from build123d import *

# Parameters (mm, degrees)
BOSS_EXTRUDE1_START    = 0.03
SKETCH1_W              = 7
SKETCH1_H              = 7
BOSS_EXTRUDE1_DEPTH    = 0.73
SKETCH2_R              = 0.478943658
CUT_EXTRUDE1_DEPTH     = 0.05
BOSS_EXTRUDE2_DEPTH    = 0.03
SKETCH4_W              = 0.5
SKETCH4_H              = 0.3
BOSS_EXTRUDE3_DEPTH    = 0.03
FILLET1_R              = 0.15
LPATTERN1_COUNT        = 3
LPATTERN1_PITCH        = 1.7
FILLET1_OF_LPATTERN1_R = 0.15
CIRPATTERN1_DEPTH      = 0.03


# Read off the part's stored shape, not the designer's step: CirPattern1
with BuildPart() as part:
    # Sketch1 → Boss-Extrude1 (new body)
    with BuildSketch(Plane.XY.offset(BOSS_EXTRUDE1_START)):
        Rectangle(SKETCH1_W, SKETCH1_H)
    extrude(amount=BOSS_EXTRUDE1_DEPTH)

    # Sketch2 → Cut-Extrude1 (cut)
    with BuildSketch(Plane.XY.offset(0.76)):
        with Locations((-2.534351737, 2.640370435)):
            Circle(SKETCH2_R)
    extrude(amount=-CUT_EXTRUDE1_DEPTH, mode=Mode.SUBTRACT)

    # Sketch3 → Boss-Extrude2 (add)
    with BuildSketch(Plane(origin=(0, 0, 0.03), x_dir=(-1, 0, 0), z_dir=(0, 0, -1))):
        Polygon((1.1, 1.4), (1.4, 1.1), (1.4, -1.4), (-1.4, -1.4), (-1.4, 1.4), align=None)
    extrude(amount=BOSS_EXTRUDE2_DEPTH)

    # Sketch4 → Boss-Extrude3 (add)
    with BuildSketch(Plane(origin=(0, 0, 0.03), x_dir=(-1, 0, 0), z_dir=(0, 0, -1))):
        with Locations((-3.25, 1.7)):
            Rectangle(SKETCH4_W, SKETCH4_H)
    boss_extrude3 = extrude(amount=BOSS_EXTRUDE3_DEPTH)

    # Fillet1
    fillet1_edges = [part.edges().sort_by_distance(p)[0] for p in [
        (3, 1.85, 0.015),
        (3, 1.55, 0.015),
    ]]
    fillet(fillet1_edges, radius=FILLET1_R - 0.0001)  # a hair under: the kernel refuses the full size

    # LPattern1: Boss-Extrude3 ×3
    with Locations(*[(0, -i * LPATTERN1_PITCH, 0) for i in range(1, LPATTERN1_COUNT)]):
        add(boss_extrude3)

    # Fillet1 of LPattern1
    fillet1_of_lpattern1_edges = [part.edges().sort_by_distance(p)[0] for p in [
        (3, 0.15, 0.015),
        (3, -0.15, 0.015),
        (3, -1.55, 0.015),
        (3, -1.85, 0.015),
    ]]
    fillet(fillet1_of_lpattern1_edges, radius=FILLET1_OF_LPATTERN1_R - 0.0001)  # a hair under: the kernel refuses the full size

    # CirPattern1 outline → CirPattern1 (add)
    with BuildSketch(Plane.XY):
        with BuildLine():
            Line((-3.5, 1.85), (-3.5, 1.55))
            Line((-3.5, 1.55), (-3.15, 1.55))
            ThreePointArc((-3.15, 1.55), (-3.043933983, 1.593933983), (-3, 1.7))
            ThreePointArc((-3, 1.7), (-3.043933983, 1.806066017), (-3.15, 1.85))
            Line((-3.15, 1.85), (-3.5, 1.85))
        make_face()
        with BuildLine():
            Line((1.55, -3.15), (1.55, -3.5))
            Line((1.55, -3.5), (1.85, -3.5))
            Line((1.85, -3.5), (1.85, -3.15))
            ThreePointArc((1.85, -3.15), (1.806066017, -3.043933983), (1.7, -3))
            ThreePointArc((1.7, -3), (1.593933983, -3.043933983), (1.55, -3.15))
        make_face()
        with BuildLine():
            Line((-0.15, -3.15), (-0.15, -3.5))
            Line((-0.15, -3.5), (0.15, -3.5))
            Line((0.15, -3.5), (0.15, -3.15))
            ThreePointArc((0.15, -3.15), (0.106066017, -3.043933983), (0, -3))
            ThreePointArc((0, -3), (-0.106066017, -3.043933983), (-0.15, -3.15))
        make_face()
        with BuildLine():
            Line((-1.85, -3.15), (-1.85, -3.5))
            Line((-1.85, -3.5), (-1.55, -3.5))
            Line((-1.55, -3.5), (-1.55, -3.15))
            ThreePointArc((-1.55, -3.15), (-1.593933983, -3.043933983), (-1.7, -3))
            ThreePointArc((-1.7, -3), (-1.806066017, -3.043933983), (-1.85, -3.15))
        make_face()
        with BuildLine():
            Line((-3.15, -1.55), (-3.5, -1.55))
            Line((-3.5, -1.55), (-3.5, -1.85))
            Line((-3.5, -1.85), (-3.15, -1.85))
            ThreePointArc((-3.15, -1.85), (-3.043933983, -1.806066017), (-3, -1.7))
            ThreePointArc((-3, -1.7), (-3.043933983, -1.593933983), (-3.15, -1.55))
        make_face()
        with BuildLine():
            Line((-3.15, 0.15), (-3.5, 0.15))
            Line((-3.5, 0.15), (-3.5, -0.15))
            Line((-3.5, -0.15), (-3.15, -0.15))
            ThreePointArc((-3.15, -0.15), (-3.043933983, -0.106066017), (-3, 0))
            ThreePointArc((-3, 0), (-3.043933983, 0.106066017), (-3.15, 0.15))
        make_face()
        with BuildLine():
            Line((1.85, 3.5), (1.55, 3.5))
            Line((1.55, 3.5), (1.55, 3.15))
            ThreePointArc((1.55, 3.15), (1.593933983, 3.043933983), (1.7, 3))
            ThreePointArc((1.7, 3), (1.806066017, 3.043933983), (1.85, 3.15))
            Line((1.85, 3.15), (1.85, 3.5))
        make_face()
        with BuildLine():
            Line((0.15, 3.5), (-0.15, 3.5))
            Line((-0.15, 3.5), (-0.15, 3.15))
            ThreePointArc((-0.15, 3.15), (-0.106066017, 3.043933983), (0, 3))
            ThreePointArc((0, 3), (0.106066017, 3.043933983), (0.15, 3.15))
            Line((0.15, 3.15), (0.15, 3.5))
        make_face()
        with BuildLine():
            Line((-1.55, 3.5), (-1.85, 3.5))
            Line((-1.85, 3.5), (-1.85, 3.15))
            ThreePointArc((-1.85, 3.15), (-1.806066017, 3.043933983), (-1.7, 3))
            ThreePointArc((-1.7, 3), (-1.593933983, 3.043933983), (-1.55, 3.15))
            Line((-1.55, 3.15), (-1.55, 3.5))
        make_face()
    extrude(amount=CIRPATTERN1_DEPTH)


solid = part.part
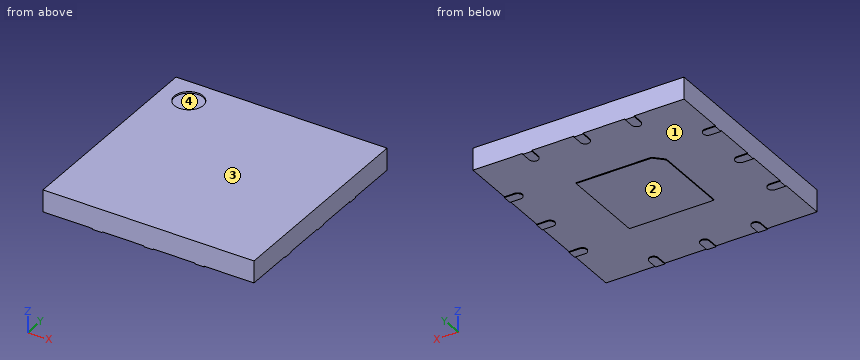
Input: part model. Units: mm. Frame: model coordinates. Face numbers are marked on the shaded views. A direction names the side the tool comes from. Coordinates: 2 decimals unless noted, no trailing zeros. Order: outer loops, then holes, each group sorted by start corner. A loop starts at its lowest first (then second) coordinate and runs counter-clockwise, first axis right, second up. Notation, with made-up numbers: M -2.5,10 L 32.5,10 A17 ccw 32.5,23 Z; hole C -28,67 d11. An arc over 180 degrees is marked long. Answer in a Markdown table with one row per item.
(1) Section query C-C, the plane x = 2. Output: boundary loops of the cut face in (y, z).
Numbers:
| item | result |
|---|---|
| outline | M -3.5,0.03 L 3.5,0.03 L 3.5,0.76 L -3.5,0.76 Z |
(2) Material intervals for line 1 (Z direction, x = 2.25, y = 1), sorted ascending. Write a range as [from, to].
Numbers:
| item | result |
|---|---|
| line 1 | z = [0.03, 0.76] |
(3) Access query for the marked faces 1 and 2. Directions: +Z, -Z, +X, -X, +Y, -Y. A direction counts if a zero-diameter tool reaches every point of the face in a straight line with its end or side. Return the directions, or none.
Numbers:
| item | result |
|---|---|
| face 1 | -Z |
| face 2 | -Z, +X, -X, +Y, -Y |
(4) Draft query along Y for the marked faces 3 and 4. Return one class per face: pulls with the +Y half, pulls with the -Y half, needs draft (parallel to the pull), parting line crosses it, or undercut.
Numbers:
| item | result |
|---|---|
| face 3 | needs draft |
| face 4 | undercut |
